Verification items for the finished model (mm, model axes). Face numbers are marked on the shaded views. A direction names the side the tool comes from. Coordinates: 2 decimals unless noted, no trailing zeros. Order: outer loops, then holes, each group sorted by start corner. A loop starts at its lowest first (then second) coordinate and runs counter-clockwise, first axis right, second up. Notation, with made-up numbers: M 0,21 L 40,21 A7 cw 40,29 Z; hole C 77.5,65 d4. An arc over 180 degrees is marked long. Return JSON: item names as keys, results as strings. Group by question number.
1. Mould release check, pull along Y, two halves, no side actions. Record for the marked faces 1, 2, 3 and 4: +Y half, -Y half, draft (parallel to the pull), parting line (faces both ways), or undercut.
2. Section check B-B, the plane y = 5.5. Record the cut outline in (x, z).
3. Material ranges on line 1 along X through (y, z) = (-30.5, 20.5); line 2 along Y through (x, z) = (-87.5, 39.5); line 3 along Z through (x, y) = (-67.5, -12), recorded low to high.
4. Section check A-A, the plane z = 22.5. Record the cut outline in (x, y).
5. Section check C-C, the plane x = 63. Record the cut outline in (y, z).
6. Set-up check for the marked faces 5 and 6: record each of +Z, -Z, +X, -X, +Y, -Y from which the full face is reachable in a straight line by a thin tool's end or side.
```python
from build123d import *

# Parameters (mm, degrees)
F0_W     = 200
F0_H     = 100
F1_DEPTH = 50
F2_T     = -2.5
F3_R     = 5


with BuildPart() as f1:
    # F0 (on Top) → F1 (new body)
    with BuildSketch(Plane.XY):
        Rectangle(F0_W, F0_H)
    extrude(amount=F1_DEPTH)

    # F2
    f2_openings = [f1.faces().sort_by_distance(p)[0] for p in [
        (0, 0, 50),
    ]]
    offset(amount=F2_T, openings=f2_openings)

    # F3
    f3_edges = [f1.edges().sort_by_distance(p)[0] for p in [
        (0, -50, 0),
        (100, 0, 0),
        (0, 50, 0),
        (-100, 0, 0),
    ]]
    fillet(f3_edges, radius=F3_R)


solid = f1.part
```
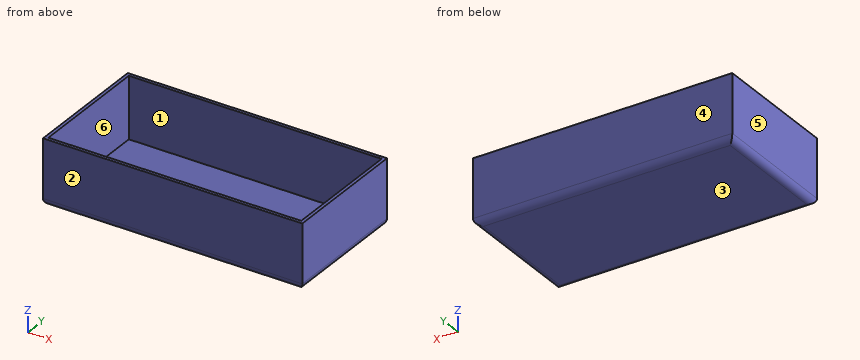
Answers follow:
{
 "1": {"face 1": "undercut", "face 2": "-Y half", "face 3": "draft", "face 4": "+Y half"},
 "2": {"outline": "M -100,5 A5 ccw -95,0 L 95,0 A5 ccw 100,5 L 100,50 L 97.5,50 L 97.5,2.5 L -97.5,2.5 L -97.5,50 L -100,50 Z"},
 "3": {"line 1": "-100 to -97.5, 97.5 to 100", "line 2": "-50 to -47.5, 47.5 to 50", "line 3": "0 to 2.5"},
 "4": {"outline": "M -100,-50 L 100,-50 L 100,50 L -100,50 Z; hole M -97.5,-47.5 L 97.5,-47.5 L 97.5,47.5 L -97.5,47.5 Z"},
 "5": {"outline": "M -50,5 A5 ccw -45,0 L 45,0 A5 ccw 50,5 L 50,50 L 47.5,50 L 47.5,2.5 L -47.5,2.5 L -47.5,50 L -50,50 Z"},
 "6": {"face 5": "+Z, -Z, -X, +Y, -Y", "face 6": "+Z"}
}
